The model under review builds one solid part; all positions refer to its coordinate system, in mm. Face numbers are marked on the shaded views. Give positions to 0.01 mm unless a question says otherwise; leave off trailing zeros. Order: outer loops, then holes, each group sorted by start corner. A loop starts at its lowest first (then second) coordinate and runs counter-clockwise, first axis right, second up. Notation, with made-up numbers: (24, -28) -> (53, -28) arc R21 ccw to (53, -11) -> close; hole circle Ø4 at (-33.75, 74.25). An arc over 180 degrees is marked (long way). Use one line per item in the form item = value.
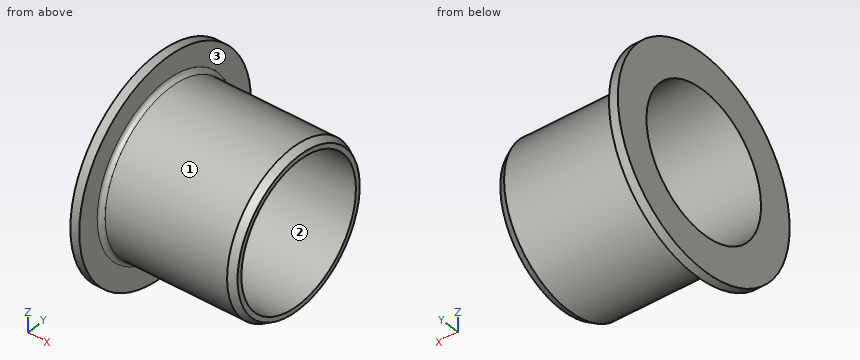
```python
from build123d import *

# Parameters (mm, degrees)
F2_SIZE2 = 0.4618802154
F2_SIZE  = 0.8
F3_R     = 0.5


with BuildPart() as f1:
    # F0 (on Front) → F1 (revolve)
    with BuildSketch(Plane.XZ):
        Polygon((0, 12), (0, 8), (1, 8), (16, 8), (16, 9), (1, 9), (1, 12), align=None)
    revolve(axis=Axis((8, 0, 0), (1, 0, 0)))

    # F2
    f2_edges = [f1.edges().sort_by_distance(p)[0] for p in [
        (16, 0, -9),
    ]]
    f2_side = f1.faces().sort_by_distance((8.5, 0, -9))[0]
    chamfer(f2_edges, length=F2_SIZE, length2=F2_SIZE2, reference=f2_side)

    # F3
    f3_edges = [f1.edges().sort_by_distance(p)[0] for p in [
        (1, 0, -9),
    ]]
    fillet(f3_edges, radius=F3_R)


solid = f1.part
```
1. The part is to be moulded in two halves that separate along Y. For the marked faces 1, 2 and 3, say which applies: +Y half, -Y half, draft (parallel to the pull), parting line (faces both ways), or undercut.
Values:
face_1 = parting line
face_2 = undercut
face_3 = draft
2. For L1, parallel to Y at x = 6.25, z = 0; L2, parallel to Y at x = 7, z = -1.25, list the stretches that pass through material, from the lowest coordinate up.
Values:
L1 = -9 to -8, 8 to 9
L2 = -8.91 to -7.9, 7.9 to 8.91
3. Add section A-A on y = 0. Give the boundary of the cut face in (x, z).
Values:
outline = (0, -12) -> (1, -12) -> (1, -9.5) arc R0.5 cw to (1.5, -9) -> (15.2, -9) -> (16, -8.54) -> (16, -8) -> (0, -8) -> close; (0, 8) -> (16, 8) -> (16, 8.54) -> (15.2, 9) -> (1.5, 9) arc R0.5 cw to (1, 9.5) -> (1, 12) -> (0, 12) -> close
4. Add section C-C on x = 3.75. Give the boundary of the cut face in (y, z), then the cut area to 3 significant figures.
Values:
outline = circle Ø18 at (0, 0); hole circle Ø16 at (0, 0)
area = 53.4 mm^2
5. For pin 1 Ø1.5 at (x, z) = (6.5, 1.5) entering from -Y; pin 2 Ø4 at (x, y) = (5.5, -2.5) entering from -Z; pin 3 Ø2 at (x, z) = (12.5, 5.5) entering from -Y, all flat-tipped, find the tip position at first contact; note any pin that passes through.
Values:
pin_1 = -8.97
pin_2 = -8.99
pin_3 = -7.79
